Build history of the part. All positions in model axes, mm. Face numbers are marked on the shaded views. A direction names the side the tool comes from. Give positions to 0.01 mm unless a question says otherwise; leave off trailing zeros. Order: outer loops, then holes, each group sorted by start corner. A loop starts at its lowest first (then second) coordinate and runs counter-clockwise, first axis right, second up. Notation, with made-up numbers: M 62,-10 L 91,-10 A20 cw 91,22 Z; hole C 74,88 d4. An arc over 180 degrees is marked long. Answer as CSV lines item,"result".
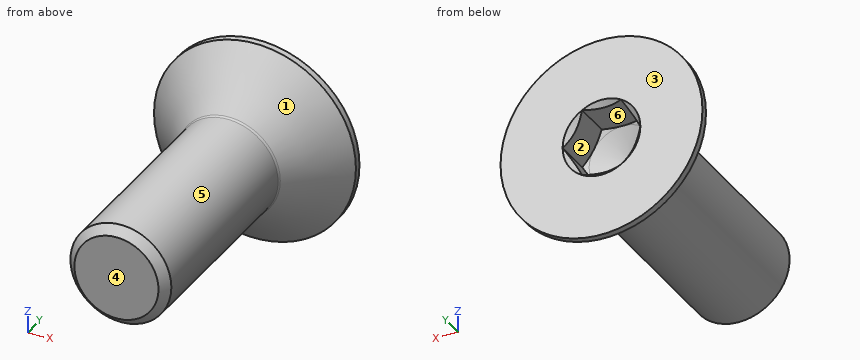
from build123d import *

# Parameters (mm, degrees)
CORTE_EXTRUS_O1_REACH = 11.055


with BuildPart() as part:
    # Esboço1 → Revolução1 (revolve)
    with BuildSketch(Plane.XY):
        with BuildLine():
            Line((0, -1.800860619), (1, -1.2))
            Line((1, -1.2), (1, 0))
            Line((1, 0), (3, 0))
            Line((3, 0), (3, -0.2))
            Line((3, -0.2), (1.529289322, -1.670710678))
            ThreePointArc((1.529289322, -1.670710678), (1.507612047, -1.703153013), (1.5, -1.741421356))
            Line((1.5, -1.741421356), (1.5, -7.75))
            Line((1.5, -7.75), (1.25, -8))
            Line((1.25, -8), (0, -8))
            Line((0, -8), (0, -1.800860619))
        make_face()
    revolve(axis=Axis((0, -1000, 0), (0, 1, 0)))

    # Corte-extrusão1: up to this cone (the profile starts inside it)
    corte_extrus_o1_end = Plane(origin=(0, 0, 0), z_dir=(0, 1, 0)).offset(-1.800859619) * Cone(1.664e-06, 27.215955714, 16.352994998, align=(Align.CENTER, Align.CENTER, Align.MIN), mode=Mode.PRIVATE)
    # Esboço2 → Corte-extrusão1 (cut, up to the surface)
    with BuildSketch(Plane(origin=(0, 0, 0), x_dir=(1, 0, 0), z_dir=(0, 1, 0)), mode=Mode.PRIVATE) as corte_extrus_o1_sk1:
        Polygon((-1.154700538, 0), (-0.577350269, -1), (0.577350269, -1), (1.154700538, 0), (0.577350269, 1), (-0.577350269, 1), align=None)
    corte_extrus_o1_tool1 = extrude(corte_extrus_o1_sk1.sketch, amount=-CORTE_EXTRUS_O1_REACH, mode=Mode.PRIVATE) & corte_extrus_o1_end
    add(corte_extrus_o1_tool1.solids().sort_by_distance((0, 0, 0))[0], mode=Mode.SUBTRACT)

    # Esboço3 → Corte-Revolução1 (revolve, cut)
    with BuildSketch(Plane.XY, mode=Mode.PRIVATE) as corte_revolu_o1_sk:
        Polygon((1.154700538, 0), (0, -1.154700538), (0, 0), align=None)
    revolve(corte_revolu_o1_sk.sketch.rotate(Axis((0, -1000, 0), (0, 1, 0)), 180), axis=Axis((0, -1000, 0), (0, 1, 0)), mode=Mode.SUBTRACT)


solid = part.part
Item 1: Probe line 1 along Y through (x, z) = (2, 0); line 2 along X through (y, z) = (-1, -0.15); line 3 along Z through (x, y) = (0, -0.5). List the from-to ranges inside material, lowest first. Write a range as from..to.
Geometry says:
line 1,"y = -1.2..0"
line 2,"x = -2.19..-1.07, 1.07..2.19"
line 3,"z = -2.7..-1, 1..2.7"
Item 2: Band-saw the part on A-A (y = -3.25). Give the cut face in (x, z).
Geometry says:
outline,"C 0,0 d3"
Item 3: 3-axis set-ups, long thin cutter, end or side, ignore diameter. For the marked faces 4, 5 and 6: which of +Z, -Z, +X, -X, +Y, -Y reach the whole face in a straight line?
Geometry says:
face 4,"+Z, -Z, +X, -X, -Y"
face 5,"-Y"
face 6,"+Y"
Item 4: Pull direction X, two halves, no side cores. Call the marked faces 1, 2 and 3: released by +X, released by -X, zero draft, split by the parting line, or undercut.
Geometry says:
face 1,"split by the parting line"
face 2,"undercut"
face 3,"zero draft"
Item 5: Drop flat-ended pins along their axis: pin 1 (1 mm diameter, centred on x = 2, z = -2.5, fed in from -Y); pin 2 (2 mm diameter, centred on x = -1, z = -1.5, fed in from +Y); pin 3 (1.5 mm diameter, centred on y = -2.5, z = -2, fed in from +X). Give the stop position or say it passes through.
Geometry says:
pin 1,"stops at y = -0.5"
pin 2,"stops at y = 0"
pin 3,"stops at x = 0.83"
